Autodesk Inventor part; units mm, degrees
ref_plane "YZ Plane" through (0, 0, 0) normal (1, 0, 0) x (0, 1, 0)
ref_plane "XZ Plane" through (0, 0, 0) normal (0, 1, 0) x (-1, 0, 0)
ref_plane "XY Plane" through (0, 0, 0) normal (0, 0, 1) x (1, 0, 0)
sketch "스케치1" plane through (0, 0, 0) normal (0, 0, 1) x (1, 0, 0)
  circle A0 centre (0, 0) radius 10
  line L0 (0, 0) -> (6, 0)
  line L1 (0, 0) -> (0, 6.1705) construction
  circle A1 centre (6, 0) radius 1.6
  circle A2 centre (-6, 0) radius 1.6
  line L2 (0, 0) -> (0, -6)
  circle A3 centre (0, -6) radius 1.6
  circle A4 centre (0, 6) radius 1.6
  dimension "d0" = 20
  dimension "d1" = 6
  dimension "d2" = 3.2
  dimension "d22" = 6
  dimension "d23" = 3.2
extrude "돌출1" add sketch "스케치1" along normal blind 35
sketch "스케치2" plane through (0, 0, 35) normal (0, 0, 1) x (1, 0, 0)
  line L0 (6, 0) -> (3.3, 0)
  line L1 (3.3, 1.5588) -> (6, 3.1177)
  line L2 (6, 3.1177) -> (8.7, 1.5588)
  line L3 (8.7, 1.5588) -> (8.7, -1.5588)
  line L4 (8.7, -1.5588) -> (6, -3.1177)
  line L5 (6, -3.1177) -> (3.3, -1.5588)
  line L6 (3.3, -1.5588) -> (3.3, 1.5588)
  line L7 (0, 6) -> (0, 3.3)
  line L8 (-1.5588, 3.3) -> (-3.1177, 6)
  line L9 (-3.1177, 6) -> (-1.5588, 8.7)
  line L10 (-1.5588, 8.7) -> (1.5588, 8.7)
  line L11 (1.5588, 8.7) -> (3.1177, 6)
  line L12 (3.1177, 6) -> (1.5588, 3.3)
  line L13 (1.5588, 3.3) -> (-1.5588, 3.3)
  line L14 (-6, 0) -> (-3.3, 0)
  line L15 (-3.3, -1.5588) -> (-6, -3.1177)
  line L16 (-6, -3.1177) -> (-8.7, -1.5588)
  line L17 (-8.7, -1.5588) -> (-8.7, 1.5588)
  line L18 (-8.7, 1.5588) -> (-6, 3.1177)
  line L19 (-6, 3.1177) -> (-3.3, 1.5588)
  line L20 (-3.3, 1.5588) -> (-3.3, -1.5588)
  line L21 (0, -6) -> (0, -3.3)
  line L22 (1.5588, -3.3) -> (3.1177, -6)
  line L23 (3.1177, -6) -> (1.5588, -8.7)
  line L24 (1.5588, -8.7) -> (-1.5588, -8.7)
  line L25 (-1.5588, -8.7) -> (-3.1177, -6)
  line L26 (-3.1177, -6) -> (-1.5588, -3.3)
  line L27 (-1.5588, -3.3) -> (1.5588, -3.3)
  point P0 (0, 0)
  point P1 (0, 6)
  point P2 (0, -6)
  dimension "d24" = 2.7
  dimension "d27" = 360
sketch "스케치3" plane through (0, 0, 0) normal (0, 0, -1) x (-1, 0, 0)
  circle A0 centre (0, 0) radius 10
  circle A1 centre (-6, 0) radius 1.6
  circle A2 centre (6, 0) radius 1.6
extrude "돌출3" cut sketch "스케치3" against normal blind 7
sketch "스케치4" plane through (0, 0, 7) normal (0, 0, -1) x (-1, 0, 0)
  circle A0 centre (0, 0) radius 10
  circle A1 centre (0, 0) radius 11.2
  dimension "d13" = 1.2
extrude "돌출4" add sketch "스케치4" against normal blind 4
chamfer "모따기2" distance 1.2 angle 45 1 edges at (-10, 0, 11)
chamfer "모따기3" distance 1.2 angle 60 1 edges at (-10, 0, 35) measured on face at (0.0643, -1.4706, 35)
extrude "돌출5" cut sketch "스케치2" against normal blind 2.8
sketch "스케치5" plane through (0, 0, 35) normal (0, 0, 1) x (1, 0, 0)
  circle A0 centre (0, 6) radius 1.6
  line L0 (1.5588, 8.7) -> (3.1177, 6)
  line L1 (-1.5588, 8.7) -> (1.5588, 8.7)
  line L2 (-3.1177, 6) -> (-1.5588, 8.7)
  line L3 (-1.5588, 3.3) -> (-3.1177, 6)
  line L4 (1.5588, 3.3) -> (-1.5588, 3.3)
  line L5 (3.1177, 6) -> (1.5588, 3.3)
  line L6 (1.5588, 8.7) -> (1.5588, 10.4142)
  line L7 (1.5588, 10.4142) -> (-1.5595, 10.4142)
  line L8 (-1.5588, 8.7) -> (-1.5588, 10.4142)
  point P0 (0, 0)
extrude "돌출6" cut sketch "스케치5" against normal blind 2.8 contours L1 L8 L7 L6
pattern_circular "원형 패턴1" count 4 over 360 about axis through (0, 0, 0) along (0, 0, 1) of "돌출6"
properties part number "Test_Shaft"
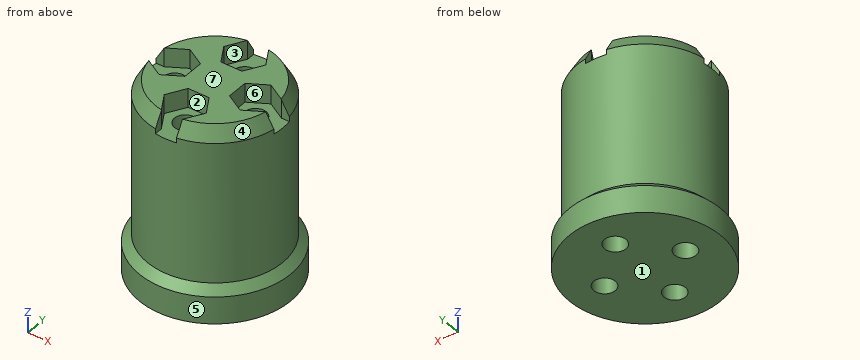
Can you work these out from the model? Positions are in its coordinate system, mm. Face numbers are marked on the shaded views. A direction names the side the tool comes from. Coordinates: 2 decimals unless noted, no trailing zeros. Write each loop counter-clockwise with the first axis right and the second up, starting at its lowest first coordinate (ties: lowest second). Pieces come first, ordered by that corner, then holes. Notation, with made-up numbers: (-16.75, 44.25) -> (-3.75, 44.25) arc R7 ccw to (-3.75, 54.25) -> close; hole circle Ø11 at (1, 27). An arc over 180 degrees is marked (long way). Write item = value, one per line.
(1) Imagine slicing it at A-A (y = 0). State how many separate pieces and enclosed holes the cut face has, and give its area (3 significant figures).
Verdict:
separate_pieces = 3
enclosed_holes = 0
area = 372 mm^2
(2) On a 3-axis mill with a long thin cutter (end or side, diameter ignored), from which of +Z, -Z, +X, -X, +Y, -Y can I reach the whole of each face in a straight line? I mean the marked faces 1, 2 and 3. Say none if no direction works.
Verdict:
face_1 = -Z, +X, -X, +Y, -Y
face_2 = +Z, -Y
face_3 = +Z
(3) For pin 1 (5 mm diameter, centred on y = 7.5, z = 22.5, fed in from -X); pin 2 (3.5 mm diameter, centred on x = 0, y = 6, fed in from +Z); pin 3 (1.5 mm diameter, centred on x = -9, y = 7, fed in from +Z), each with a flat end and sliding along its axis, tell me the tip position at first contact or that it passes through.
Verdict:
pin_1 = -8.66
pin_2 = 32.2
pin_3 = 11.55
(4) If I drill on probe 1 along X at (y, z) = (0, 18.5); probe 2 along Y at (x, z) = (-0.75, 23), over which ranges is the centre line in solid material (lowest first)?
Verdict:
probe_1 = -10 to -7.6, -4.4 to 4.4, 7.6 to 10
probe_2 = -9.97 to -7.41, -4.59 to 4.59, 7.41 to 9.97
(5) Imagine slicing it at C-C (z = 12.75). Please give me the cut outline in (x, y), and give its area (3 significant figures).
Verdict:
outline = circle Ø20 at (0, 0); hole circle Ø3.2 at (-6, 0); hole circle Ø3.2 at (0, -6); hole circle Ø3.2 at (0, 6); hole circle Ø3.2 at (6, 0)
area = 282 mm^2
(6) Imagine slicing it at D-D (z = 9.5). Please give me the cut outline in (x, y).
Verdict:
outline = circle Ø22.4 at (0, 0); hole circle Ø3.2 at (-6, 0); hole circle Ø3.2 at (0, -6); hole circle Ø3.2 at (0, 6); hole circle Ø3.2 at (6, 0)
(7) Thinking about a two-plate mould opening in X: for the marked faces 4, 5, 6 and 7, which applies, +X half, -X half, draft (parallel to the pull), parting line (faces both ways), or undercut?
Verdict:
face_4 = +X half
face_5 = parting line
face_6 = undercut
face_7 = draft
